```python
from build123d import *

# Parameters (mm, degrees)
ESQUISSE2_W             = 2
ESQUISSE2_H             = 12.833084331
ENL_V_MAT_EXTRU_1_DEPTH = 1.5


with BuildPart() as part:
    # Esquisse1 → Révolution1 (revolve)
    with BuildSketch(Plane.XY):
        Polygon((0, 0), (0, 5), (3.5, 5), (3.5, 3), (10.5, 3), (10.5, 2.25), (14.5, 2.25), (15, 1.75), (15, 0), align=None)
    revolve(axis=Axis((15, 0, 0), (-1, 0, 0)))

    # Esquisse2 → Enlèv. mat.-Extru.1 (cut)
    with BuildSketch(Plane.ZY):
        with Locations((0, -0.051559527)):
            Rectangle(ESQUISSE2_W, ESQUISSE2_H)
    extrude(amount=-ENL_V_MAT_EXTRU_1_DEPTH, mode=Mode.SUBTRACT)


solid = part.part
```
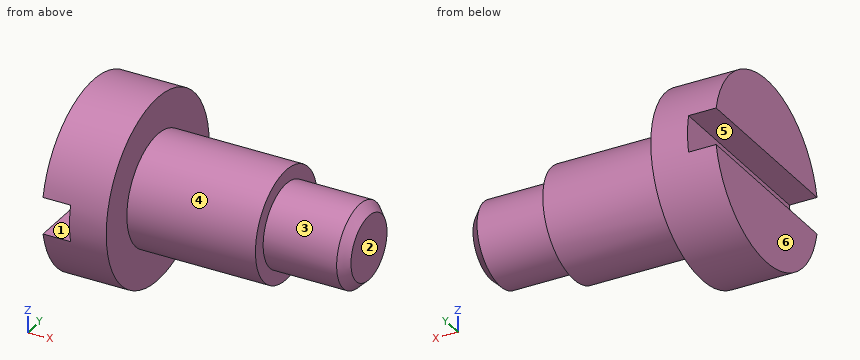
CAD build for the part. Positions are in the model's coordinates, mm. Face numbers are marked on the shaded views. A direction names the side the tool comes from. Round coordinates to 2 decimals unless told otherwise and drop trailing zeros. Write each loop counter-clockwise with the first axis right and the second up, starting at its lowest first coordinate (ties: lowest second). Pieces come first, ordered by that corner, then holes. Notation, with made-up numbers: (54, 68) -> (112, 68) arc R10 cw to (112, 86) -> close; hole circle Ø2 at (-21.5, 61). An arc over 180 degrees is marked (long way). Answer in a Markdown table with one row per item. Add a question column.
Item 1: Drop flat-ended pins along their axis: pin 1 Ø1.2 at (x, y) = (1, -1) entering from +Z; pin 2 Ø1 at (y, z) = (1, -3.5) entering from -X; pin 3 Ø2 at (x, y) = (2.5, 4) entering from +Z; pin 4 Ø1 at (x, y) = (7.5, -1) entering from +Z. Give the stop position or say it passes through.
Item 2: Saw through at A-A, the plane y = 0. Write the cut outline in (x, z), then the cut area to 3 significant figures.
Item 3: Saw through at B-B, the plane z = 0. Write the cut outline in (x, y), then the cut area to 3 significant figures.
Item 4: Mould opens along Z. For the marked faces 4, 5 and 6 say: pulls with the +Z half, pulls with the -Z half, needs draft (parallel to the pull), parting line crosses it, or undercut.
Item 5: Saw through at C-C, the plane x = 7.75. Write the cut outline in (y, z).
Item 6: Saw through at D-D, the plane y = -4. Write the cut outline in (x, z).
Item 7: Drill centre lines: line 1 (X direction, y = -4, z = 0.5); line 2 (X direction, y = -2.25, z = -3.5); line 3 (Z direction, x = 1, y = -1.75). Where is each one in solid material? Low to high. Write a range as from..to.
Item 8: Which spindle directions (+Z, -Z, +X, -X, +Y, -Y) get a long thin tool onto all of the face, cutting with end or side? Do the marked faces 1, 2 and 3. Say none if no direction does.
Findings below:
| question | item | result |
|---|---|---|
| 1 | pin 1 | stops at z = 4.98 |
| 1 | pin 2 | stops at x = 0 |
| 1 | pin 3 | stops at z = 4 |
| 1 | pin 4 | stops at z = 2.96 |
| 2 | outline | (0, -5) -> (3.5, -5) -> (3.5, -3) -> (10.5, -3) -> (10.5, -2.25) -> (14.5, -2.25) -> (15, -1.75) -> (15, 1.75) -> (14.5, 2.25) -> (10.5, 2.25) -> (10.5, 3) -> (3.5, 3) -> (3.5, 5) -> (0, 5) -> (0, 1) -> (1.5, 1) -> (1.5, -1) -> (0, -1) -> close |
| 2 | area | 94.0 mm^2 |
| 3 | outline | (1.5, -5) -> (3.5, -5) -> (3.5, -3) -> (10.5, -3) -> (10.5, -2.25) -> (14.5, -2.25) -> (15, -1.75) -> (15, 1.75) -> (14.5, 2.25) -> (10.5, 2.25) -> (10.5, 3) -> (3.5, 3) -> (3.5, 5) -> (1.5, 5) -> close |
| 3 | area | 82.0 mm^2 |
| 4 | face 4 | parting line crosses it |
| 4 | face 5 | undercut |
| 4 | face 6 | needs draft |
| 5 | outline | circle Ø6 at (0, 0) |
| 6 | outline | (0, -3) -> (3.5, -3) -> (3.5, 3) -> (0, 3) -> (0, 1) -> (1.5, 1) -> (1.5, -1) -> (0, -1) -> close |
| 7 | line 1 | x = 1.5..3.5 |
| 7 | line 2 | x = 0..3.5 |
| 7 | line 3 | z = -4.68..-1, 1..4.68 |
| 8 | face 1 | -X, +Y, -Y |
| 8 | face 2 | +Z, -Z, +X, +Y, -Y |
| 8 | face 3 | +X |
